For this review, take the finished solid that the model builds, in its own axes (mm). Give positions to 0.01 mm unless a question says otherwise; leave off trailing zeros. Write each loop counter-clockwise with the first axis right and the second up, starting at its lowest first coordinate (ties: lowest second). Pieces come first, ordered by that corner, then holes. Notation, with made-up numbers: (37.25, 86.25) -> (45.25, 86.25) arc R16 cw to (45.25, 116.25) -> close; hole circle Ø5 at (23, -8.5). An arc over 180 degrees is marked (long way). Write item = value, one per line.
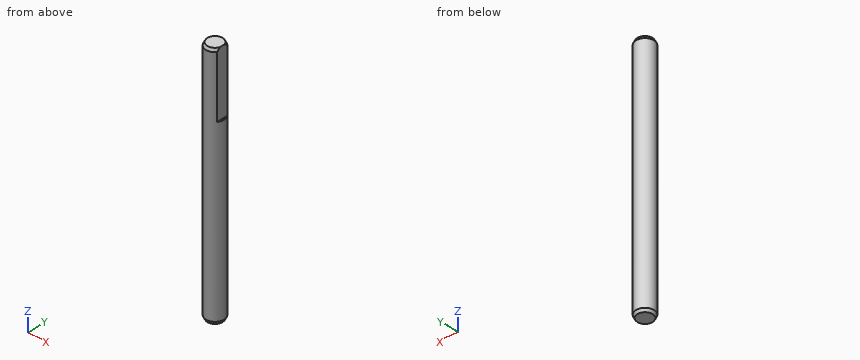
```python
from build123d import *

# Parameters (mm, degrees)
SKETCH012_R      = 2.5
PAD006_DEPTH     = 68
POCKET003_DEPTH  = 18
CHAMFER002_SIZE2 = 0.4
CHAMFER002_SIZE  = 0.8


with BuildPart() as part:
    # Sketch012 → Pad006 (new body)
    with BuildSketch(Plane.XY):
        Circle(SKETCH012_R)
    extrude(amount=PAD006_DEPTH)

    # Sketch013 (on Face3 of Pad006) → Pocket003 (cut)
    with BuildSketch(Plane.XY.offset(68)):
        with BuildLine():
            ThreePointArc((2, -1.5), (2.5, 0), (2, 1.5))
            Line((2, 1.5), (2, -1.5))
        make_face()
    extrude(amount=-POCKET003_DEPTH, mode=Mode.SUBTRACT)

    # Chamfer002
    chamfer002_edges = [part.edges().sort_by_distance(p)[0] for p in [
        (-2.5, 0, 68),
        (-2.5, 0, 0),
    ]]
    chamfer002_side = part.faces().sort_by_distance((-2.5, 0, 34))[0]
    chamfer(chamfer002_edges, length=CHAMFER002_SIZE, length2=CHAMFER002_SIZE2, reference=chamfer002_side)


with BuildPart() as part_1:
    # Body003 placement: moved
    add(part.part.moved(Location((0, 0, 2.8))))


solid = part_1.part
```
(1) To check wall thickness, follow probe 1 along Y at (x, z) = (0.2, 50); probe 2 along X at (y, z) = (-0.1, 40); probe 3 along X at (y, z) = (0.8, 56). State the ranges of each line that lie inside material, in increasing order.
Answers below:
probe_1 = -2.49 to 2.49
probe_2 = -2.5 to 2.5
probe_3 = -2.37 to 2
(2) For pin 1 (1.5 mm diameter, centred on y = 0, z = 64, fed in from +X); pin 2 (1.5 mm diameter, centred on y = -2, z = 54.5, fed in from -X); pin 3 (1.5 mm diameter, centred on x = -2, z = 23.5, fed in from -Y), all flat-tipped, find the tip position at first contact; note any pin that passes through.
Answers below:
pin_1 = 2
pin_2 = -2.17
pin_3 = -2.17
(3) Take a section at A-A (y = 0). Write out the cut boundary in (x, z).
Answers below:
outline = (-2.5, 3.6) -> (-2.1, 2.8) -> (2.1, 2.8) -> (2.5, 3.6) -> (2.5, 52.8) -> (2, 52.8) -> (2, 70.8) -> (-2.1, 70.8) -> (-2.5, 70) -> close
(4) Take a section at C-C (z = 66). Write out the cut boundary in (x, y), plus the area to 3 significant figures.
Answers below:
outline = (2, -1.5) -> (2, 1.5) arc R2.5 ccw (long way) to start
area = 18.6 mm^2
(5) Take a section at B-B (z = 15.5). Write out the cut boundary in (x, y), plus the area to 3 significant figures.
Answers below:
outline = circle Ø5 at (0, 0)
area = 19.6 mm^2
